Build history of the part. All positions in model axes, mm. Round coordinates to 2 decimals unless told otherwise and drop trailing zeros. Write each loop counter-clockwise with the first axis right and the second up, starting at its lowest first coordinate (ties: lowest second). Pieces come first, ordered by that corner, then holes. Notation, with made-up numbers: (21.25, 50.25) -> (57.25, 50.25) arc R23 cw to (57.25, 72.25) -> close; hole circle Ø4 at (-37, 35.5). An arc over 180 degrees is marked (long way). Return JSON: item names as keys, results as strings.
from build123d import *

# Parameters (mm, degrees)
SKETCH1_R           = 16.916621232
BOSS_EXTRUDE1_DEPTH = 64
SKETCH2_W           = 106.262974488
SKETCH2_H           = 38.987679284
BOSS_EXTRUDE2_DEPTH = 10


with BuildPart() as part:
    # Sketch1 → Boss-Extrude1 (new body)
    with BuildSketch(Plane(origin=(0, 0, 0), x_dir=(1, 0, 0), z_dir=(0, 1, 0))):
        with Locations((22.72979363, -8.239550191)):
            Circle(SKETCH1_R)
    extrude(amount=BOSS_EXTRUDE1_DEPTH)

    # Sketch2 → Boss-Extrude2 (add)
    with BuildSketch(Plane(origin=(0, 64, 0), x_dir=(1, 0, 0), z_dir=(0, 1, 0))):
        with Locations((22.72979363, -8.239550191)):
            Rectangle(SKETCH2_W, SKETCH2_H)
    extrude(amount=BOSS_EXTRUDE2_DEPTH)


solid = part.part
Q1. Pin check, flat tips, straight feed: pin 1 Ø19.5 at (x, z) = (16.5, 14.5) entering from -Y; pin 2 Ø2 at (x, z) = (50.5, -5) entering from -Y; pin 3 Ø2 at (y, z) = (41.5, -3) entering from +X; pin 4 Ø3 at (y, z) = (55.5, 7) entering from +X. Stop position of each tip, or through.
Verdict:
{"pin 1": "stops at y = 0", "pin 2": "stops at y = 64", "pin 3": "stops at x = 36.2", "pin 4": "stops at x = 39.65"}
Q2. Saw through at C-C on z = -5.5. List the corners of the cut face in (x, y), then the cut area to 3 significant figures.
Verdict:
{"outline": "(-30.4, 64) -> (12.86, 64) -> (12.86, 0) -> (32.6, 0) -> (32.6, 64) -> (75.86, 64) -> (75.86, 74) -> (-30.4, 74) -> close", "area": "2,330 mm²"}
Q3. Saw through at D-D on y = 13. List the corners of the cut face in (x, z), then the cut area to 3 significant figures.
Verdict:
{"outline": "circle Ø33.83 at (22.73, 8.24)", "area": "899 mm²"}
Q4. Saw through at B-B on x = 3. List the corners of the cut face in (y, z).
Verdict:
{"outline": "(64, -11.25) -> (74, -11.25) -> (74, 27.73) -> (64, 27.73) -> close"}
Q5. Two-plate mould, pull along Y, no slides. Class faces 1 (the flat face through (22, 74, 8)), 2 (the flat face through (22, 0, 8)), 3 (the cylindrical face through (38.865, 31.552, 3.158)): +Y half, -Y half, draft (parallel to the pull), parting line (faces both ways), or undercut.
Verdict:
{"face 1": "+Y half", "face 2": "-Y half", "face 3": "draft"}
Q6. Saw through at A-A on z = 1. List the corners of the cut face in (x, y), then the cut area to 3 significant figures.
Verdict:
{"outline": "(-30.4, 64) -> (7.44, 64) -> (7.44, 0) -> (38.02, 0) -> (38.02, 64) -> (75.86, 64) -> (75.86, 74) -> (-30.4, 74) -> close", "area": "3,020 mm²"}
Q7. Wall check: L1, parallel to Y at x = -18, z = 20.5; L2, parallel to X at y = 52, z = 8; L3, parallel to X at y = 37, z = 23. Give the ranges that are in metal, low to high.
Verdict:
{"L1": "y = 64 to 74", "L2": "x = 5.81 to 39.64", "L3": "x = 14.47 to 30.99"}
